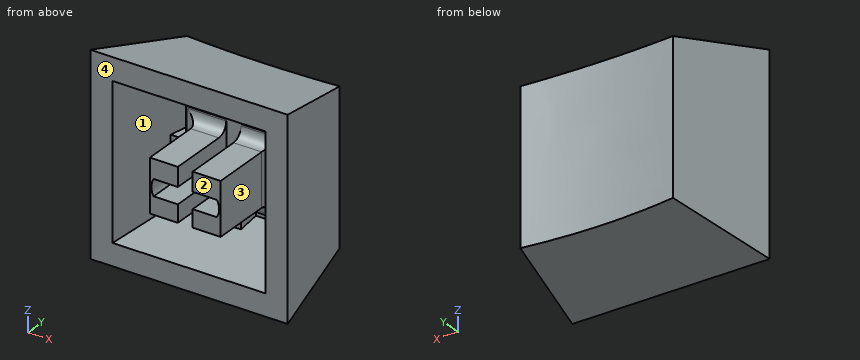
```python
from build123d import *

# Parameters (mm, degrees)
SHELL1_T                = -2
SKETCH5_W               = 1.35
SKETCH5_H               = 12.225319986
SKETCH5_W_2             = 12.114403326
SKETCH5_H_2             = 1.35
BOSS_EXTRUDE1_DEPTH     = 4
CUT_EXTRUDE3_DEPTH      = 10
CUT_EXTRUDE3_DEPTH_BACK = 10
BOSS_EXTRUDE2_START     = -0.5
BOSS_EXTRUDE2_DEPTH     = 10
BOSS_EXTRUDE2_2_DEPTH   = 10
SKETCH8_W               = 8.738759906
SKETCH8_H               = 7.199411956
SKETCH8_W_2             = 6.5
SKETCH8_H_2             = 4.831184338
BOSS_EXTRUDE4_DEPTH     = 2
FILLET4_R               = 1


with BuildPart() as part:
    # Loft1: read off the stored shape, not the designer's step
    # Loft1: loft between two sections, ruled curve by curve
    loft1_from = [
        Edge.make_line((-9.05, 0, 9.05), (-9.05, 0, -9.05)),
        Edge.make_line((-9.05, 0, -9.05), (9.05, 0, -9.05)),
        Edge.make_line((9.05, 0, 9.05), (-9.05, 0, 9.05)),
        Edge.make_line((9.05, 0, -9.05), (9.05, 0, 9.05)),
    ]
    loft1_to = [
        Edge.make_line((-7, 10, 6.318777005), (-7, 10, -7.681222995)),
        Edge.make_line((-7, 10, -7.681222995), (7, 10, -7.681222995)),
        Edge.make_line((7, 10, 6.318777005), (-7, 10, 6.318777005)),
        Edge.make_line((7, 10, -7.681222995), (7, 10, 6.318777005)),
    ]
    loft1 = Solid(Shell([*[Face.make_surface_from_curves(loft1_from[k], loft1_to[k]) for k in range(4)], Face(Wire(loft1_from)), Face(Wire(loft1_to))]))
    add(loft1)

    # Shell1
    shell1_openings = [part.faces().sort_by_distance(p)[0] for p in [
        (0, 0, 0),
    ]]
    offset(amount=SHELL1_T, openings=shell1_openings, kind=Kind.INTERSECTION)

    # Sketch5 → Boss-Extrude1 (add)
    with BuildSketch(Plane(origin=(0, 10, 0), x_dir=(1, 0, 0), z_dir=(0, 1, 0))):
        with Locations((0, 0.862108036)):
            Rectangle(SKETCH5_W, SKETCH5_H)
        with Locations((0.109128691, 0.681416915)):
            Rectangle(SKETCH5_W_2, SKETCH5_H_2)
    extrude(amount=-BOSS_EXTRUDE1_DEPTH)

    # Sketch4 → Cut-Extrude3 (cut, two sides: drawn at the far end of the back side and taken through both)
    with BuildSketch(Plane.XY.offset(-CUT_EXTRUDE3_DEPTH_BACK)):
        with BuildLine():
            Line((-7, 10), (7, 10))
            add(Edge.make_bspline(
                [(-7, 10), (-2.602300298, 9.460265696), (1.993912061, 9.41154423), (7, 10)],
                knots=[0, 0, 0, 0, 1, 1, 1, 1], degree=3))
        make_face()
    extrude(amount=CUT_EXTRUDE3_DEPTH + CUT_EXTRUDE3_DEPTH_BACK, mode=Mode.SUBTRACT)



with BuildPart() as body_2:
    # Sketch6 → Boss-Extrude2 (new body)
    with BuildSketch(Plane(origin=(0, 10, 0), x_dir=(1, 0, 0), z_dir=(0, 1, 0)).offset(BOSS_EXTRUDE2_START)):
        with BuildLine():
            Line((0.675, -0.005353557), (0.675, -1.75))
            Line((0.675, -1.75), (3.25, -1.75))
            Line((3.25, -1.75), (3.25, 3.09053704))
            Line((3.25, 3.09053704), (0.675, 3.09053704))
            Line((0.675, 3.09053704), (0.675, 1.494646443))
            Line((0.675, 1.494646443), (2.90473751, 1.494646443))
            ThreePointArc((2.90473751, 1.494646443), (3.109676589, 0.744646443), (2.90473751, -0.005353557))
            Line((2.90473751, -0.005353557), (0.675, -0.005353557))
        make_face()
    extrude(amount=-BOSS_EXTRUDE2_DEPTH)


with BuildPart() as body_3:
    # Sketch6 → Boss-Extrude2 2 (new body)
    with BuildSketch(Plane(origin=(0, 10, 0), x_dir=(1, 0, 0), z_dir=(0, 1, 0)).offset(BOSS_EXTRUDE2_START)):
        with BuildLine():
            Line((-0.675, -1.75), (-0.675, -0.005353557))
            Line((-0.675, -0.005353557), (-2.90473751, -0.005353557))
            ThreePointArc((-2.90473751, -0.005353557), (-3.109676589, 0.744646443), (-2.90473751, 1.494646443))
            Line((-2.90473751, 1.494646443), (-0.675, 1.494646443))
            Line((-0.675, 1.494646443), (-0.675, 3.09053704))
            Line((-0.675, 3.09053704), (-3.25, 3.09053704))
            Line((-3.25, 3.09053704), (-3.25, -1.75))
            Line((-3.25, -1.75), (-0.675, -1.75))
        make_face()
    extrude(amount=-BOSS_EXTRUDE2_2_DEPTH)


with BuildPart() as part_1:
    add(part.part)

    add(body_2.part)  # Boss-Extrude4 merges body 2

    add(body_3.part)  # Boss-Extrude4 merges body 3
    # Sketch8 → Boss-Extrude4 (add)
    with BuildSketch(Plane(origin=(0, 8, -8), x_dir=(1, 0, 0), z_dir=(0, -1, 0))):
        with Locations((0, 7.325055129)):
            Rectangle(SKETCH8_W, SKETCH8_H)
        with Locations((0, 7.325055129)):
            Rectangle(SKETCH8_W_2, SKETCH8_H_2, mode=Mode.SUBTRACT)
    extrude(amount=BOSS_EXTRUDE4_DEPTH)

    # Fillet4
    fillet4_edges = [part_1.edges().sort_by_distance(p)[0] for p in [
        (3.25, 6, -0.67026852),
        (-3.25, 6, -0.67026852),
        (-1.9625, 6, -3.09053704),
        (1.9625, 6, -3.09053704),
        (1.9625, 6, 1.75),
        (-1.9625, 6, 1.75),
    ]]
    fillet(fillet4_edges, radius=FILLET4_R)


solid = part_1.part
```
CAD build for the part. Positions are in the model's coordinates, mm. Face numbers are marked on the shaded views. A direction names the side the tool comes from. Give positions to 0.01 mm unless a question says otherwise; leave off trailing zeros. Return JSON: item names as keys, results as strings. Group by question number.
(1) Flat gauge pins, fed straight in: pin 1 Ø2 at (x, y) = (-4.5, 8.5) entering from +Z; pin 2 Ø5 at (x, y) = (-5.5, 9) entering from -Z; pin 3 Ø1 at (y, z) = (7.5, 1.5) entering from -X (3 decimals). Where does each tip first touch, or does it go through?
(2) Band-saw the part on A-A (y = 5.5). State how many separate pieces and enclosed holes the cut face has, and give its area (3 significant figures).
(3) 3-axis set-ups, long thin cutter, end or side, ignore diameter. For the marked faces 1 and 2: which of +Z, -Z, +X, -X, +Y, -Y reach the whole face in a straight line?
(4) Drill centre lines: L1, parallel to X at y = 5.75, z = -2 (3 decimals); L2, parallel to Z at x = -1, y = 1.25; L3, parallel to X at y = 6.75, z = -2.5. Where is each one in solid material? Low to high. Write a range as [from, to].
(5) Mould opens along Z. For the marked faces 3 and 4 say: pulls with the +Z half, pulls with the -Z half, needs draft (parallel to the pull), parting line crosses it, or undercut.
Entries:
{
 "1": {"pin 1": "stops at z = 7", "pin 2": "stops at z = -8.16", "pin 3": "stops at x = -7.615"},
 "2": {"separate pieces": "3", "enclosed holes": "1", "area": "133 mm^2"},
 "3": {"face 1": "-Y", "face 2": "+Z, -Z, +X, -X, -Y"},
 "4": {"L1": "x = [-7.871, -5.83], [-3.589, -0.675], [0.675, 3.589], [5.83, 7.871]", "L2": "z = [-8.88, -6.86], [-3.09, -1.49], [0.01, 1.75], [6.64, 8.71]", "L3": "x = [-7.67, -5.62], [-4.37, 4.37], [5.62, 7.67]"},
 "5": {"face 3": "undercut", "face 4": "needs draft"}
}
